Verification items for the finished model (mm, model axes). A direction names the side the tool comes from. Give positions to 0.01 mm unless a question says otherwise; leave off trailing zeros. Order: outer loops, then holes, each group sorted by start corner. A loop starts at its lowest first (then second) coordinate and runs counter-clockwise, first axis right, second up.
(1) Sectioned sample at C-C on y = -10.5. Record the cut outline in (x, z), plus the area to 3 significant figures.
(2) Sectioned sample at B-B on z = 0. Record the cut outline in (x, y).
(3) Scan lines: L1, parallel to Y at x = -15.5, z = 20.15; L2, parallel to Z at x = 6, y = 7.5; L3, parallel to Y at x = 6, z = -3.5. Record each from-to range of solid material in increasing order.
(4) Access from +Z, -Z, +X, -X, +Y, -Y to the whole of each face (thin tool, end or side, straight path). Record for faces 1 (the face through (15, 24, 0)), 2 (the face through (-21, -24, 21)), 3 (the face through (-15, 24, 0)), 4 (the face through (21, -24, 21)).
(5) Sectioned sample at A-A on x = 0. Record the cut outline in (y, z).
(6) Sectioned sample at D-D on x = -19. Record the cut outline in (y, z), plus the area to 3 significant figures.
(7) Mould release check, pull along Y, two halves, no side actions. Record for faces 5 (the face through (16.77, -42.47, 20.96)), 6 (the face through (-19.4, 17.7, -0.3)), 7 (the face through (0, -47, 21)), 8 (the face through (24, -1, 0)): pulls with the +Y half, pulls with the -Y half, needs draft (parallel to the pull), parting line crosses it, or undercut.
(8) Gauge pin test, flat ends, axial feed: pin 1 (2 mm diameter, centred on x = 16.5, z = 14.5, fed in from +Y); pin 2 (5 mm diameter, centred on y = -27.5, z = 20, fed in from -X); pin 3 (2.5 mm diameter, centred on x = 15.5, y = -41.5, fed in from -Z); pin 4 (1.8 mm diameter, centred on y = -15, z = 21, fed in from +X). Record the tip position at first contact, or that the pin passes through.
```python
from build123d import *

# Parameters (mm, degrees)
BOSS_EXTRUDE1_DEPTH      = 55
BOSS_EXTRUDE1_DEPTH_BACK = 5
SKETCH1_W                = 48
SKETCH1_H                = 48
SKETCH2_R                = 7.6
CUT_EXTRUDE1_DEPTH       = 77.843997814
SKETCH3_R                = 7.6
CUT_EXTRUDE2_DEPTH       = 77.843997814
SKETCH6_W                = 42
SKETCH6_H                = 42
BOSS_EXTRUDE2_DEPTH      = 6
SKETCH7_R                = 1.6
CUT_EXTRUDE4_DEPTH       = 74.246160309
CUT_EXTRUDE5_DEPTH       = 77.843997814
CHAMFER12_SIZE           = 5
CHAMFER12_SIZE_2         = 10
CHAMFER13_SIZE           = 10
CHAMFER13_SIZE_2         = 5
CHAMFER14_SIZE           = 3
CHAMFER15_SIZE           = 5


with BuildPart() as part:
    # Sketch1 → Boss-Extrude1 (new, two sides: drawn at the far end of the back side and taken through both)
    with BuildSketch(Plane(origin=(0, 0, 0), x_dir=(1, 0, 0), z_dir=(0, 1, 0)).offset(-BOSS_EXTRUDE1_DEPTH_BACK)):
        Rectangle(SKETCH1_W, SKETCH1_H)
    extrude(amount=BOSS_EXTRUDE1_DEPTH + BOSS_EXTRUDE1_DEPTH_BACK)

    # Sketch2 → Cut-Extrude1 (cut, through all)
    with BuildSketch(Plane.XY.offset(24)):
        with Locations((0, 28)):
            Circle(SKETCH2_R)
    extrude(amount=-CUT_EXTRUDE1_DEPTH, mode=Mode.SUBTRACT)

    # Sketch3 → Cut-Extrude2 (cut, through all)
    with BuildSketch(Plane(origin=(24, 0, 0), x_dir=(0, 0, -1), z_dir=(1, 0, 0))):
        with Locations((0, 7)):
            Circle(SKETCH3_R)
    extrude(amount=-CUT_EXTRUDE2_DEPTH, mode=Mode.SUBTRACT)

    # Sketch6 → Boss-Extrude2 (add)
    with BuildSketch(Plane.XY.offset(24)):
        with Locations((0, -26)):
            Rectangle(SKETCH6_W, SKETCH6_H)
    extrude(amount=-BOSS_EXTRUDE2_DEPTH)

    # Sketch7 → Cut-Extrude4 (cut, through all)
    with BuildSketch(Plane(origin=(0, 0, 18), x_dir=(-1, 0, 0), z_dir=(0, 0, -1))):
        with Locations((-15.5, -10.5)):
            Circle(SKETCH7_R)
        with Locations((-15.5, -41.5)):
            Circle(SKETCH7_R)
        with Locations((15.5, -41.5)):
            Circle(SKETCH7_R)
        with Locations((15.5, -10.5)):
            Circle(SKETCH7_R)
    extrude(amount=-CUT_EXTRUDE4_DEPTH, mode=Mode.SUBTRACT)

    # Sketch9 → Cut-Extrude5 (cut, through all)
    with BuildSketch(Plane(origin=(0, 0, -24), x_dir=(-1, 0, 0), z_dir=(0, 0, -1))):
        with BuildLine():
            Line((-15, 28), (-15, 20.4))
            Line((-15, 20.4), (-24, 20.4))
            Line((-24, 20.4), (-24, 55))
            Line((-24, 55), (24, 55))
            Line((24, 55), (24, 20.4))
            Line((24, 20.4), (15, 20.4))
            Line((15, 20.4), (15, 28))
            ThreePointArc((15, 28), (0, 43), (-15, 28))
        make_face()
    extrude(amount=-CUT_EXTRUDE5_DEPTH, mode=Mode.SUBTRACT)

    # Chamfer12
    # the kernel refuses this chamfer: 10, 5 mm, written as the material it takes off along each edge
    with BuildSketch(Plane(origin=(24, 20.4, -49.898288738), x_dir=(0.06891834360170909, -0.9976223042390326, 0), z_dir=(0, 0, 1))) as chamfer12_piece_1_section:
        Polygon((CHAMFER12_SIZE * 0.997622304239, -CHAMFER12_SIZE * 0.0689183436017), (-CHAMFER12_SIZE_2 * 0.0689183436017, -CHAMFER12_SIZE_2 * 0.997622304239), (0, 0), align=None)
    chamfer12_piece_1 = extrude(amount=99.796577476, mode=Mode.PRIVATE)
    chamfer12_piece_1 = split(chamfer12_piece_1, bisect_by=Plane(origin=(15, 18.773620907, 0), z_dir=(1, 0, 0)), keep=Keep.TOP, mode=Mode.PRIVATE)
    add(chamfer12_piece_1, mode=Mode.SUBTRACT)

    # Chamfer13
    # the kernel refuses this chamfer: 10, 5 mm, written as the material it takes off along each edge
    with BuildSketch(Plane(origin=(-24, 20.4, -49.898288738), x_dir=(0.9998508956747119, 0.017268075123668212, 0), z_dir=(0, 0, 1))) as chamfer13_piece_1_section:
        Polygon((CHAMFER13_SIZE * 0.999850895675, -CHAMFER13_SIZE * 0.0172680751237), (-CHAMFER13_SIZE_2 * 0.0172680751237, -CHAMFER13_SIZE_2 * 0.999850895675), (0, 0), align=None)
    chamfer13_piece_1 = extrude(amount=99.796577476, mode=Mode.PRIVATE)
    chamfer13_piece_1 = split(chamfer13_piece_1, bisect_by=Plane(origin=(-15, 18.773620907, 0), z_dir=(-1, 0, 0)), keep=Keep.TOP, mode=Mode.PRIVATE)
    add(chamfer13_piece_1, mode=Mode.SUBTRACT)

    # Chamfer14
    chamfer14_edges = [part.edges().sort_by_distance(p)[0] for p in [
        (-24, -5, 0),
        (24, -5, 0),
    ]]
    chamfer(chamfer14_edges, length=CHAMFER14_SIZE)

    # Chamfer15
    chamfer15_edges = [part.edges().sort_by_distance(p)[0] for p in [
        (-21, -47, 21),
        (21, -47, 21),
    ]]
    chamfer(chamfer15_edges, length=CHAMFER15_SIZE)


solid = part.part
```
Ans:
1. outline: (-21, 18) - (-17.1, 18) - (-17.1, 24) - (-21, 24) - close; (-13.9, 18) - (13.9, 18) - (13.9, 24) - (-13.9, 24) - close; (17.1, 18) - (21, 18) - (21, 24) - (17.1, 24) - close
1. area: 214 mm2
2. outline: (-24, -2) - (-21, -5) - (21, -5) - (24, -2) - (24, -0.6) - (-24, -0.6) - close; (-24, 14.6) - (24, 14.6) - (24, 15.4) - (15, 19.9) - (15, 28) arc R15 ccw to (-15, 28) - (-15, 19.9) - (-24, 15.4) - close; hole circle Ø15.2 at (0, 28)
3. L1: y = -47 to -43.1, -39.9 to -12.1, -8.9 to 19.65
3. L2: z = -24 to -7.58, 7.58 to 24
3. L3: y = -5 to 0.25, 13.75 to 23.34, 32.66 to 41.75
4. face 1: +Z, -Z, +X, +Y
4. face 2: +Z, -Z, -X, -Y
4. face 3: +Z, -Z, -X, +Y
4. face 4: +Z, -Z, +X, -Y
5. outline: (-47, 18) - (-5, 18) - (-5, -24) - (20.4, -24) - (20.4, 24) - (-47, 24) - close; (35.6, -24) - (43, -24) - (43, 24) - (35.6, 24) - close; hole circle Ø15.2 at (7, 0)
6. outline: (-44, 18) - (-5, 18) - (-5, -24) - (17.9, -24) - (17.9, 24) - (-44, 24) - close; hole circle Ø15.2 at (7, 0)
6. area: 1,150 mm2
7. face 5: undercut
7. face 6: pulls with the +Y half
7. face 7: pulls with the -Y half
7. face 8: needs draft
8. pin 1: stops at y = 19.65
8. pin 2: stops at x = -21
8. pin 3: passes through
8. pin 4: stops at x = 21
